Input: part model. Units: mm. Frame: model coordinates. A direction names the side the tool comes from. Give positions to 0.01 mm unless a question says otherwise; leave off trailing zeros. Loops run counter-clockwise (first coordinate to the right, second up) from the corner with the lowest first, then second, coordinate; pieces in that order, holes last. Notation, with made-up numbers: (64, -39.75) -> (93, -39.75) arc R19 cw to (93, -8.75) -> close; hole circle Ø7 at (-39.5, 89). An arc over 180 degrees is marked (long way). Answer as a JSON object with one key per item and string values.
```python
from build123d import *

# Parameters (mm, degrees)
F1_DEPTH  = 3
F3_DEPTH  = 0.5
F5_DEPTH  = 3.01
F6_SIZE2  = 3
F6_SIZE   = 2
F7_R      = 2
F8_R      = 4.25
F9_DEPTH  = 0.2
F10_R     = 4.045
F11_DEPTH = 0.2
F12_W     = 15.3
F12_H     = 81.59
F12_W_2   = 25
F12_H_2   = 73.2
F13_DEPTH = 25


with BuildPart() as f1:
    # F0 (on Top) → F1 (new body)
    with BuildSketch(Plane.XY):
        Polygon((-86.6, 48.4397485852), (-90, 48.4397485852), (-90, -36.7602514148), (-50.005, -70.7602514148), (50.005, -70.7602514148), (90, -36.7602514148), (90, 48.4397485852), (86.6, 48.4397485852), (86.6, 47.3397485852), (-86.6, 47.3397485852), align=None)
    extrude(amount=F1_DEPTH)

    # F2 (on face) → F3 (cut)
    with BuildSketch(Plane.XY.offset(3)):
        Polygon((28.905, 18.6197485852), (28.905, 47.3397485852), (28.405, 47.3397485852), (28.405, 19.1197485852), (23.595, 19.1197485852), (23.595, 4.3397485852), (28.405, 4.3397485852), (28.405, -16.1802514148), (23.595, -16.1802514148), (23.595, -41.8302514148), (28.405, -41.8302514148), (28.405, -58.7802514148), (23.595, -58.7802514148), (23.595, -70.7602514148), (24.095, -70.7602514148), (24.095, -59.2802514148), (28.405, -59.2802514148), (28.405, -71.6557353735), (28.905, -71.7005729675), (28.905, -59.2802514148), (67.82, -59.2802514148), (67.82, -35.9962806106), (67.32, -35.9962806106), (67.32, -58.7802514148), (28.905, -58.7802514148), (28.905, -41.3302514148), (24.095, -41.3302514148), (24.095, -16.6802514148), (28.905, -16.6802514148), (28.905, 4.8397485852), (24.095, 4.8397485852), (24.095, 18.6197485852), align=None)
        Polygon((-28.405, 19.1197485852), (-28.405, 47.3397485852), (-28.905, 47.3397485852), (-28.905, 18.6197485852), (-24.095, 18.6197485852), (-24.095, 4.8397485852), (-28.905, 4.8397485852), (-28.905, -16.6802514148), (-24.095, -16.6802514148), (-24.095, -41.3302514148), (-28.905, -41.3302514148), (-28.905, -58.7802514148), (-28.905, -59.2802514148), (-28.405, -59.2802514148), (-24.095, -59.2802514148), (-24.095, -70.7602514148), (-23.595, -70.7602514148), (-23.595, -58.7802514148), (-28.405, -58.7802514148), (-28.405, -41.8302514148), (-23.595, -41.8302514148), (-23.595, -16.1802514148), (-28.405, -16.1802514148), (-28.405, 4.3397485852), (-23.595, 4.3397485852), (-23.595, 19.1197485852), align=None)
        Polygon((-28.905, -59.2802514148), (-28.905, -58.7802514148), (-67.32, -58.7802514148), (-67.32, -35.9962806106), (-67.82, -35.9962806106), (-67.82, -59.2802514148), align=None)
    extrude(amount=-F3_DEPTH, mode=Mode.SUBTRACT)

    # F4 (on face) → F5 (join)
    with BuildSketch(Plane.XY.offset(3)):
        with BuildLine():
            Line((14.115, 7.3147485852), (-14.115, 7.3147485852))
            ThreePointArc((-14.115, 7.3147485852), (-16.971711396, 6.1314599812), (-18.155, 3.2747485852))
            Line((-18.155, 3.2747485852), (-18.155, -29.6952514148))
            ThreePointArc((-18.155, -29.6952514148), (-16.971711396, -32.5519628108), (-14.115, -33.7352514148))
            Line((-14.115, -33.7352514148), (14.115, -33.7352514148))
            ThreePointArc((14.115, -33.7352514148), (16.971711396, -32.5519628108), (18.155, -29.6952514148))
            Line((18.155, -29.6952514148), (18.155, 3.2747485852))
            ThreePointArc((18.155, 3.2747485852), (16.971711396, 6.1314599812), (14.115, 7.3147485852))
        make_face()
    extrude(amount=F5_DEPTH)

    # F6
    f6_edges = [f1.edges().sort_by_distance(p)[0] for p in [
        (-18.155, -13.210251, 6.01),
    ]]
    f6_side = f1.faces().sort_by_distance((0, -13.210251, 6.01))[0]
    chamfer(f6_edges, length=F6_SIZE, length2=F6_SIZE2, reference=f6_side)

    # F7
    f7_edges = [f1.edges().sort_by_distance(p)[0] for p in [
        (15.557498, 4.717246, 6.01),
    ]]
    fillet(f7_edges, radius=F7_R)

    # F8 (on face) → F9 (join)
    with BuildSketch(Plane.XY.offset(6.01)):
        with Locations((0, -13.2102514148)):
            Circle(F8_R)
    extrude(amount=F9_DEPTH)

    # F10 (on face) → F11 (join)
    with BuildSketch(Plane.XY.offset(3)):
        with Locations((-12.63, -50.5702514148)):
            Circle(F10_R)
        with Locations((12.63, -50.5702514148)):
            Circle(F10_R)
    extrude(amount=F11_DEPTH)

    # F12 (on face) → F13 (cut)
    with BuildSketch(Plane.XY.offset(3)):
        with Locations((-77.54, 2.8447485852)):
            Rectangle(F12_W, F12_H)
        with Locations((77.54, 2.8447485852)):
            Rectangle(F12_W, F12_H)
        with Locations((-42.955, -21.1302514148)):
            Rectangle(F12_W_2, F12_H_2)
        with Locations((42.955, -21.1302514148)):
            Rectangle(F12_W_2, F12_H_2)
    extrude(amount=-F13_DEPTH, mode=Mode.SUBTRACT)


solid = f1.part
```
Q1. Section D-D, the plane x = -79. Return the cut outline in (y, z), then the cut area to 3 significant figures.
Evaluation:
{"outline": "(-46.11, 0) -> (-37.95, 0) -> (-37.95, 3) -> (-46.11, 3) -> close; (43.64, 0) -> (47.34, 0) -> (47.34, 3) -> (43.64, 3) -> close", "area": "35.6 mm2"}
Q2. Access query for faces 5 (the flat face through (-70.282, -53.522, 1.479)), 6 (the flat face through (13, -51, 3.2)), 7 (the flat face through (19, -11, 3)). Directions: +Z, -Z, +X, -X, +Y, -Y. A direction counts if a zero-diameter tool reaches every point of the face in a straight line with its end or side. Return the directions, or none.
Evaluation:
{"face 5": "+Z, -Z, -X, -Y", "face 6": "+Z, +X, -X, -Y", "face 7": "+Z"}
Q3. Section B-B, the plane z = 1.5. Return the cut outline in (x, y) (3 decimals).
Evaluation:
{"outline": "(-90, -36.76) -> (-50.005, -70.76) -> (50.005, -70.76) -> (90, -36.76) -> (90, 48.44) -> (86.6, 48.44) -> (86.6, 47.34) -> (-86.6, 47.34) -> (-86.6, 48.44) -> (-90, 48.44) -> close; hole (-85.19, -37.95) -> (-69.89, -37.95) -> (-69.89, 43.64) -> (-85.19, 43.64) -> close; hole (-55.455, -57.73) -> (-30.455, -57.73) -> (-30.455, 15.47) -> (-55.455, 15.47) -> close; hole (30.455, -57.73) -> (55.455, -57.73) -> (55.455, 15.47) -> (30.455, 15.47) -> close; hole (69.89, -37.95) -> (85.19, -37.95) -> (85.19, 43.64) -> (69.89, 43.64) -> close"}
Q4. Section A-A, the plane x = -34.5. Return the cut outline in (y, z).
Evaluation:
{"outline": "(-70.76, 0) -> (-57.73, 0) -> (-57.73, 3) -> (-58.78, 3) -> (-58.78, 2.5) -> (-59.28, 2.5) -> (-59.28, 3) -> (-70.76, 3) -> close; (15.47, 0) -> (47.34, 0) -> (47.34, 3) -> (15.47, 3) -> close"}
Q5. Ray query, line 1 along X through (y, z) = (-4, 1) (3 decimals); line 2 along X through (y, z) = (-54, 0.5) (3 decimals); line 3 along Z through (x, y) = (-64, 14). Return the intervals inside material, ascending.
Evaluation:
{"line 1": "x = -90 to -85.19, -69.89 to -55.455, -30.455 to 30.455, 55.455 to 69.89, 85.19 to 90", "line 2": "x = -69.72 to -55.455, -30.455 to 30.455, 55.455 to 69.72", "line 3": "z = 0 to 3"}
Q6. Draft query along X for faces 1 (the conical face through (16.346, -31.976, 4.284)), 2 (the conical face through (-16.346, 5.555, 4.284)), 3 (the flat face through (28.75, -11.43, 2.5)), 4 (the flat face through (26, -65, 3)). Return one class per face: +X half, -X half, draft (parallel to the pull), parting line (faces both ways), or undercut.
Evaluation:
{"face 1": "+X half", "face 2": "-X half", "face 3": "undercut", "face 4": "draft"}
Q7. Pin query (flat end, axial travel): pin 1 (0.6 mm diameter, centred on x = 25.5, z = 3, fed in from +Y); pin 2 (6.5 mm diameter, centred on x = -14, y = -52, fed in from +Z); pin 3 (3 mm diameter, centred on x = -24, y = -44.5, fed in from +Z). Return the tip coordinate at first contact, or that it passes through.
Evaluation:
{"pin 1": "stops at y = 47.34", "pin 2": "stops at z = 3.2", "pin 3": "stops at z = 3"}
